```python
from build123d import *

# Parameters (mm, degrees)
SKETCH1_R        = 8
BODY_DEPTH       = 2.5
BODY_DEPTH_BACK  = 2.5
SKETCH3_R        = 4
BORE_HOLE_DEPTH  = 6
SKETCH4_R        = 6.5
SKETCH4_R_2      = 5
DECORATION_DEPTH = 0.3


with BuildPart() as part:
    # Sketch1 → Body (new body, two sides)
    with BuildSketch(Plane.XY) as body_sk:
        Circle(SKETCH1_R)
    extrude(amount=BODY_DEPTH)
    extrude(body_sk.sketch, amount=-BODY_DEPTH_BACK)

    # Sketch3 → Bore-Hole (cut, through all)
    with BuildSketch(Plane.XY.offset(2.5)):
        Circle(SKETCH3_R)
    extrude(amount=-BORE_HOLE_DEPTH, mode=Mode.SUBTRACT)

    # Sketch4 → Decoration (cut)
    with BuildSketch(Plane.XY.offset(2.5)):
        Circle(SKETCH4_R)
        Circle(SKETCH4_R_2, mode=Mode.SUBTRACT)
    decoration = extrude(amount=-DECORATION_DEPTH, mode=Mode.SUBTRACT)

    # Mirror1: Decoration across plane
    add(decoration.mirror(Plane.XY), mode=Mode.SUBTRACT)


solid = part.part
```
Read the model definition and answer for the solid it produces. Units are mm, in the model's axes. Give positions to 0.01 mm unless a question says otherwise; leave off trailing zeros. Write each loop counter-clockwise with the first axis right and the second up, starting at its lowest first coordinate (ties: lowest second). Pieces come first, ordered by that corner, then holes. Notation, with made-up numbers: M 45,-22.5 L 73,-22.5 A10 ccw 73,-4.5 Z; hole C 57.25,43 d6. An arc over 180 degrees is marked long. Put each result on its own line as item: value. Start each with the question number.
1. The part is cut by section A-A, the plane y = 0. Give the vertices of the cut face in (x, z).
2. The part is cut by section C-C, the plane z = 1.75. Give the vertices of the cut face in (x, y).
3. Each of these flat-tipped pins is pushed along its axis until it touches: pin 1 Ø4 at (x, y) = (0.5, 0.5) entering from +Z; pin 2 Ø2 at (x, z) = (4.5, 0.5) entering from +Y. Where does it stop, or does it pass through?
4. Consider line 1 along Y through (x, z) = (0, 2.4); line 2 along Y through (x, z) = (0, -0.5); line 3 along Z through (x, y) = (-1.25, -5.25). Determine where each line is inside the solid, lowest interval first.
5. For a pull along X with two mould halves and no side action, classify faces 1 (the flat face through (0, 7, 2.5)), 2 (the flat face through (2, -5, 2.2)), 3 (the cylindrical face through (-1.73, -7.81, 0.04)), 4 (the flat face through (2, -5, -2.2)) as released by +X, released by -X, zero draft, split by the parting line, or undercut.
6. The part is cut by section D-D, the plane y = -6. Give the vertices of the cut face in (x, z).
Final values:
1. outline: M -8,-2.5 L -6.5,-2.5 L -6.5,-2.2 L -5,-2.2 L -5,-2.5 L -4,-2.5 L -4,2.5 L -5,2.5 L -5,2.2 L -6.5,2.2 L -6.5,2.5 L -8,2.5 Z; M 4,-2.5 L 5,-2.5 L 5,-2.2 L 6.5,-2.2 L 6.5,-2.5 L 8,-2.5 L 8,2.5 L 6.5,2.5 L 6.5,2.2 L 5,2.2 L 5,2.5 L 4,2.5 Z
2. outline: C 0,0 d16; hole C 0,0 d8
3. pin 1: passes through
3. pin 2: stops at y = 7.19
4. line 1: y = -8 to -6.5, -5 to -4, 4 to 5, 6.5 to 8
4. line 2: y = -8 to -4, 4 to 8
4. line 3: z = -2.2 to 2.2
5. face 1: zero draft
5. face 2: undercut
5. face 3: split by the parting line
5. face 4: undercut
6. outline: M -5.29,-2.5 L -2.5,-2.5 L -2.5,-2.2 L 2.5,-2.2 L 2.5,-2.5 L 5.29,-2.5 L 5.29,2.5 L 2.5,2.5 L 2.5,2.2 L -2.5,2.2 L -2.5,2.5 L -5.29,2.5 Z
